Could you check a few things on this model? Use its own coordinates, in mm. A direction names the side the tool comes from. Give positions to 0.01 mm unless a question says otherwise; leave off trailing zeros. Order: outer loops, then holes, each group sorted by start corner. A loop starts at its lowest first (then second) coordinate and runs counter-clockwise, first axis right, second up. Notation, with made-up numbers: (18, -11) - (72, -11) arc R28 cw to (72, 12) - close; hole circle Ø3 at (80, 4.5). An arc over 180 degrees is marked (long way). Put each result on its own line as item: value.
from build123d import *

# Parameters (mm, degrees)
BOSS_EXTRUDE1_DEPTH = 50
SHELL1_T            = -3


with BuildPart() as part:
    # Sketch1 → Boss-Extrude1 (new body)
    with BuildSketch(Plane(origin=(0, 0, 0), x_dir=(1, 0, 0), z_dir=(0, 1, 0))):
        Polygon((-25.019, 12.954), (-25.019, -25.908), (-62.103, -25.908), (-62.103, -63.754), (39.243, -63.754), (37.465, 12.954), align=None)
    extrude(amount=BOSS_EXTRUDE1_DEPTH)

    # Shell1
    shell1_openings = [part.faces().sort_by_distance(p)[0] for p in [
        (-11.43, 25, 63.754),
    ]]
    offset(amount=SHELL1_T, openings=shell1_openings, kind=Kind.INTERSECTION)


solid = part.part
1) Which directions (+Z, -Z, +X, -X, +Y, -Y) give clear straight access to the entire face, cutting with the end or side of a thin tool? Please do faces 5 (the flat face through (7, 25, -9.954)), 6 (the flat face through (-43, 25, 25.908)), 7 (the flat face through (-1, 0, 25)).
Filled in:
face 5: +Z
face 6: -Z, -X, +Y, -Y
face 7: +Z, -Z, +X, -X, -Y
2) If I drill on line 1 (Y direction, x = 22.5, z = 31); line 2 (Z direction, x = 19.5, y = 45.5); line 3 (Z direction, x = -36, y = 30.5), over which ranges is the centre line in solid material (lowest first)? Write a range as [from, to].
Filled in:
line 1: y = [0, 3], [47, 50]
line 2: z = [-12.95, -9.95]
line 3: z = [25.91, 28.91]
3) Suppose I cut it at B-B, the plane x = -7. List the corners of the cut face in (y, z) for me.
Filled in:
outline: (0, -12.95) - (50, -12.95) - (50, 63.75) - (47, 63.75) - (47, -9.95) - (3, -9.95) - (3, 63.75) - (0, 63.75) - close
4) Suppose I cut it at D-D, the plane z = 10. List the corners of the cut face in (x, y) for me, and give its area (3 significant figures).
Filled in:
outline: (-25.02, 0) - (38, 0) - (38, 50) - (-25.02, 50) - close; hole (-22.02, 3) - (35, 3) - (35, 47) - (-22.02, 47) - close
area: 642 mm^2
5) Suppose I cut it at C-C, the plane y = 28. List the corners of the cut face in (x, z) for me (3 decimals).
Filled in:
outline: (-62.103, 25.908) - (-25.019, 25.908) - (-25.019, -12.954) - (37.465, -12.954) - (39.243, 63.754) - (36.242, 63.754) - (34.534, -9.954) - (-22.019, -9.954) - (-22.019, 28.908) - (-59.103, 28.908) - (-59.103, 63.754) - (-62.103, 63.754) - close
6) Suppose I cut it at A-A, the plane z = 33.5. List the corners of the cut face in (x, y) for me, and give its area (3 significant figures).
Filled in:
outline: (-62.1, 0) - (38.54, 0) - (38.54, 50) - (-62.1, 50) - close; hole (-59.1, 3) - (35.54, 3) - (35.54, 47) - (-59.1, 47) - close
area: 868 mm^2
7) I'm going to push flat-ended pins straight in: pin 1 (10 mm diameter, centred on x = 24, y = 9.5, fed in from +Z); pin 2 (12 mm diameter, centred on y = 31, z = 16.5, fed in from -X); pin 3 (8 mm diameter, centred on x = 19, z = 32, fed in from -Y); pin 4 (1 mm diameter, centred on x = -27, y = 30.5, fed in from +Z). Where does each tip first touch, or does it pass through?
Filled in:
pin 1: stops at z = -9.95
pin 2: stops at x = -25.02
pin 3: stops at y = 0
pin 4: stops at z = 28.91
8) We'd pull the mould along X, two halves only. Please class faces 1 (the flat face through (-40, 25, 28.908)), 2 (the flat face through (-1, 50, 25)), 3 (the flat face through (-25.019, 25, 6)), 4 (the flat face through (-22.019, 25, 9)): pulls with the +X half, pulls with the -X half, needs draft (parallel to the pull), parting line crosses it, or undercut.
Filled in:
face 1: undercut
face 2: needs draft
face 3: pulls with the -X half
face 4: undercut
